```python
from build123d import *

# Parameters (mm, degrees)
SKETCH1_W         = 45
SKETCH1_H         = 24
PUMP_BODY_DEPTH   = 33
OUTLET_START      = 33
SKETCH2_R         = 3.75
OUTLET_DEPTH      = 10
OUTLET_BORE_START = 43
SKETCH3_R         = 2.25
OUTLET_BORE_DEPTH = 15
INLET_SLOTS_START = 12
SKETCH4_W         = 2.5
SKETCH4_H         = 8
INLET_SLOTS_DEPTH = 2
CABLE_STUB_START  = -37.5
SKETCH5_R         = 2
CABLE_STUB_DEPTH  = 15


with BuildPart() as part:
    # Sketch1 → Pump_Body (new body)
    with BuildSketch(Plane(origin=(0, 0, 0), x_dir=(1, 0, 0), z_dir=(0, 1, 0))):
        Rectangle(SKETCH1_W, SKETCH1_H)
    extrude(amount=PUMP_BODY_DEPTH)

    # Sketch2 → Outlet (add)
    with BuildSketch(Plane(origin=(0, 0, 0), x_dir=(1, 0, 0), z_dir=(0, 1, 0)).offset(OUTLET_START)):
        with Locations(Location((15, 0, 0), (0, 0, 270))):
            Circle(SKETCH2_R)
    extrude(amount=OUTLET_DEPTH)

    # Sketch3 → Outlet_Bore (cut)
    with BuildSketch(Plane(origin=(0, 0, 0), x_dir=(1, 0, 0), z_dir=(0, 1, 0)).offset(OUTLET_BORE_START)):
        with Locations(Location((15, 0, 0), (0, 0, 270))):
            Circle(SKETCH3_R)
    extrude(amount=-OUTLET_BORE_DEPTH, mode=Mode.SUBTRACT)

    # Sketch4 → Inlet_Slots (cut)
    with BuildSketch(Plane.XY.offset(INLET_SLOTS_START)):
        with Locations((-14.5, 6)):
            Rectangle(SKETCH4_W, SKETCH4_H)
        with Locations((-9.5, 6)):
            Rectangle(SKETCH4_W, SKETCH4_H)
        with Locations((-4.5, 6)):
            Rectangle(SKETCH4_W, SKETCH4_H)
        with Locations((0.5, 6)):
            Rectangle(SKETCH4_W, SKETCH4_H)
    extrude(amount=-INLET_SLOTS_DEPTH, mode=Mode.SUBTRACT)

    # Sketch5 → Cable_Stub (add)
    with BuildSketch(Plane(origin=(0, 0, 0), x_dir=(0, 0, -1), z_dir=(1, 0, 0)).offset(CABLE_STUB_START)):
        with Locations((0, 22)):
            Circle(SKETCH5_R)
    extrude(amount=CABLE_STUB_DEPTH)


solid = part.part
```
The model under review builds one solid part; all positions refer to its coordinate system, in mm. A direction names the side the tool comes from. Give positions to 0.01 mm unless a question says otherwise; leave off trailing zeros. Loops run counter-clockwise (first coordinate to the right, second up) from the corner with the lowest first, then second, coordinate; pieces in that order, holes last. Notation, with made-up numbers: (5, 15.25) -> (22, 15.25) arc R34 cw to (22, 47.25) -> close; hole circle Ø2 at (8, 26.25). An arc over 180 degrees is marked (long way). Use CSV: the item, a comma, the result in double quotes.
1. Machinability: for faces 1 (the face through (-30.105, 20.226, -0.923)), 2 (the face through (15, 28, 0)), 3 (the face through (-15, 6, 10)), which of the approach directions +Z, -Z, +X, -X, +Y, -Y give a long, thin tool a straight path to every point of the face, cutting with its end or side? Answer none if there is none.
Result:
face 1,"-X"
face 2,"+Y"
face 3,"+Z"
2. To check wall thickness, follow probe 1 along X at (y, z) = (39.5, 0); probe 2 along X at (y, z) = (32, 0); probe 3 along Y at (x, z) = (-10.5, 10.75). State the ranges of each line that lie inside material, in increasing order. Write a range as from..to.
Result:
probe 1,"x = 11.25..12.75, 17.25..18.75"
probe 2,"x = -22.5..12.75, 17.25..22.5"
probe 3,"y = 0..2, 10..33"
3. Consider section C-C, the plane x = 15. Write out the cut boundary in (y, z), then the cut area to 4 significant figures.
Result:
outline,"(0, -12) -> (33, -12) -> (33, -3.75) -> (43, -3.75) -> (43, -2.25) -> (28, -2.25) -> (28, 2.25) -> (43, 2.25) -> (43, 3.75) -> (33, 3.75) -> (33, 12) -> (0, 12) -> close"
area,"799.5 mm²"
4. Consider section B-B, the plane y = 6. Write out the cut boundary in (x, z), then the cut area to 3 significant figures.
Result:
outline,"(-22.5, -12) -> (22.5, -12) -> (22.5, 12) -> (1.75, 12) -> (1.75, 10) -> (-0.75, 10) -> (-0.75, 12) -> (-3.25, 12) -> (-3.25, 10) -> (-5.75, 10) -> (-5.75, 12) -> (-8.25, 12) -> (-8.25, 10) -> (-10.75, 10) -> (-10.75, 12) -> (-13.25, 12) -> (-13.25, 10) -> (-15.75, 10) -> (-15.75, 12) -> (-22.5, 12) -> close"
area,"1,060 mm²"
5. Consider section A-A, the plane z = 0. Write out the cut boundary in (x, y), then the cut area to 3 significant figures.
Result:
outline,"(-37.5, 20) -> (-22.5, 20) -> (-22.5, 0) -> (22.5, 0) -> (22.5, 33) -> (18.75, 33) -> (18.75, 43) -> (17.25, 43) -> (17.25, 28) -> (12.75, 28) -> (12.75, 43) -> (11.25, 43) -> (11.25, 33) -> (-22.5, 33) -> (-22.5, 24) -> (-37.5, 24) -> close"
area,"1,550 mm²"
6. For P1, Ø12, axis at x = -30.5, y = 23.5, coming from the +Z side; P2, Ø8, axis at x = -8.5, y = 38.5, coming from the +Z side; P3, Ø10, axis at x = -15, z = -0.5, coming from the +Y side; P4, Ø1.6, axis at y = 7.5, z = 11, coming from the -X side, all flat-tipped, find the tip position at first contact; note any pin that passes through.
Result:
P1,"stops at z = 2"
P2,"passes through"
P3,"stops at y = 33"
P4,"stops at x = -22.5"
7. The part is to be moulded in two halves that separate along X. For faces 4 (the face through (-37.5, 22, 0)), 5 (the face through (0, 0, 0)), 6 (the face through (-0.75, 6, 11)), say which applies: +X half, -X half, draft (parallel to the pull), parting line (faces both ways), or undercut.
Result:
face 4,"-X half"
face 5,"draft"
face 6,"undercut"
8. Consider section D-D, the plane y = 36. Write out the cut boundary in (x, z).
Result:
outline,"circle Ø7.5 at (15, 0); hole circle Ø4.5 at (15, 0)"
